Source: CAD feature listing. Evaluate the final solid. Frame: model axes, mm. A direction names the side the tool comes from. Round coordinates to 2 decimals unless told otherwise and drop trailing zeros. Loops run counter-clockwise (first coordinate to the right, second up) from the corner with the lowest first, then second, coordinate; pieces in that order, holes last. Notation, with made-up numbers: M 56,-19 L 101,-19 A12 ccw 101,2 Z; hole C 85.25,58 d6. An arc over 180 degrees is marked long. Answer as a JSON object with one key per item and string values.
Autodesk Inventor part; units mm, degrees
ref_plane "YZ Plane" through (0, 0, 0) normal (1, 0, 0) x (0, 1, 0)
ref_plane "XZ Plane" through (0, 0, 0) normal (0, 1, 0) x (-1, 0, 0)
ref_plane "XY Plane" through (0, 0, 0) normal (0, 0, 1) x (1, 0, 0)
sketch "Эскиз1" plane through (0, 0, 0) normal (0, 1, 0) x (-1, 0, 0)
  line L0 (-3.5, 0) -> (-3.5, -76)
  line L1 (0, 0) -> (0, -2)
  line L2 (0, -2) -> (0, -1)
  line L3 (0, -72) -> (0, -73)
  line L4 (0, 0) -> (0, -12)
  line L5 (0, -12) -> (8, -12)
  line L6 (8, -12) -> (56, -12)
  line L7 (56, -12) -> (62, -12)
  line L8 (62, -12) -> (62, -1)
  line L9 (62, -1) -> (0, -1)
  line L10 (0, -73) -> (62, -73)
  line L11 (62, -73) -> (62, -12)
  line L12 (0, -72) -> (62, -72)
  line L13 (0, -2) -> (62, -2)
  line L14 (3.5, -76) -> (3.5, 0)
  line L15 (0, 0) -> (3, 0)
  line L16 (3, 0) -> (3, 0.6)
  line L17 (56, -12) -> (68, -12)
  line L18 (68, -12) -> (73, -12)
  line L19 (8, -12) -> (10, -12)
  circle A0 centre (10, -12) radius 1.1
  circle A1 centre (68, -12) radius 1.1
  circle A2 centre (3, 0.6) radius 1.1
  circle A3 centre (3, 0.6) radius 3
  circle A4 centre (4, -76) radius 1.1
  circle A5 centre (4, -76) radius 3.5
  line L20 (7.5, -76) -> (7.5, -73)
  line L21 (0.5, -76) -> (0.5, -73)
  line L22 (0, -73) -> (-3.5, -73)
  line L23 (6, 0.6) -> (6, -1)
  line L24 (0, -1) -> (-3.5, -1)
  line L25 (62, -73) -> (73, -73)
  line L26 (73, -73) -> (73, -1)
  line L27 (73, -1) -> (62, -1)
  line L28 (62, -1) -> (62, -73)
  line L29 (0, 0.6) -> (0, 0)
  point P0 (3.5, -73)
  point P1 (0.0606, 0)
  dimension "d6" = 2
  dimension "d7" = 1
  dimension "d8" = 1
  dimension "d9" = 12
  dimension "d10" = 8
  dimension "d11" = 48
  dimension "d12" = 6
  dimension "d39" = 3
  dimension "d40" = 0.6
  dimension "d41" = 12
  dimension "d42" = 5
  dimension "d43" = 2
  dimension "d44" = 2.2
  dimension "d45" = 2.2
  dimension "d46" = 2.2
  dimension "d47" = 6
  dimension "d48" = 2.2
  dimension "d49" = 7
extrude "Выдавливание1" add sketch "Эскиз1" along normal blind 2 contours L24 L1 L4 L5 L14 L12 L3 L22 L0 | L9 A3 L13 L1 | L1 L15 A3 L9 | L3 L12 L14 A5 L10 | L29 A3 L15 | L13 A3 L14 L5 L4 | A3 L15 A2 L14 L9 | L9 L14 L13 A3 | L10 A5 L21 | A3 L9 L14 A2 L15 | L13 L14 A3 | L9 A3 L13 L14 | L14 L5 L6 A0 L7 L11 L12 | L12 L11 L10 A5 L14 | A5 L14 L10 | L10 A5 | L23 L9 A3 | L14 A3 L13 L8 L7 L6 A0 L5 | L13 A3 L14 | L9 L8 L13 A3 | L11 L17 A1 L18 L26 L25 | A5 L10 L14 | A5 L10 L20 | L8 L27 L26 L18 A1 L17
sketch "Эскиз2" plane through (0, 2, 0) normal (0, 1, 0) x (1, 0, 0)
  line L0 (-73, 1) -> (-6, 1)
  line L1 (3.5, 1) -> (3.5, 73)
  line L2 (-73, 1) -> (3.5, 1)
  line L3 (3.5, 1) -> (3.5, 2)
  line L4 (3.5, 2) -> (-73, 2)
  line L5 (-73, 2) -> (-73, 1)
  line L6 (-7.5, 73) -> (-73, 73)
  line L7 (-73, 73) -> (3.5, 73)
  line L8 (3.5, 73) -> (3.5, 72)
  line L9 (3.5, 72) -> (-73, 72)
  line L10 (-73, 72) -> (-73, 73)
  line L11 (0, 1) -> (3.5, 1)
  line L12 (3.5, 73) -> (1.5, 73)
  line L13 (1.5, 73) -> (1.5, 1)
  line L14 (1.5, 1) -> (3.5, 1)
  line L15 (3.5, 1) -> (3.5, 73)
  point P0 (-62, 73)
  point P1 (1.5, 72)
  point P2 (1.5, 2)
  dimension "d50" = 1
  dimension "d51" = 1
  dimension "d52" = 2
extrude "Выдавливание2" add sketch "Эскиз2" along normal blind 6
sketch "Эскиз3" plane through (-62, 0, -1) normal (0, 0, 1) x (1, 0, 0)
  line L0 (65.5, 8) -> (-11, 8)
  line L1 (65.5, 8) -> (43.5, 8)
  line L2 (63.5, 8) -> (54.5, 8)
  line L3 (54.5, 8) -> (54.5, 5)
  circle A0 centre (54.5, 5) radius 1.5
  line L4 (-11, 2) -> (63.5, 2)
  line L5 (43.5, 8) -> (-11, 2)
  line L6 (-11, 2) -> (-11, 8)
  line L7 (43.5, 8) -> (-11, 8)
  point P0 (65.5, 2)
  dimension "d53" = 22
  dimension "d54" = 9
  dimension "d55" = 3
  dimension "d56" = 3
extrude "Выдавливание3" cut sketch "Эскиз3" against normal blind 76
sketch "Эскиз4" plane through (0, 8, 0) normal (0, 1, 0) x (1, 0, 0)
  circle A0 centre (-3, -0.6) radius 1.1
  circle A1 centre (-3, -0.6) radius 2.1
  dimension "d57" = 4.2
extrude "Выдавливание4" cut sketch "Эскиз4" against normal blind 6 contours A0 | A1
chamfer "Фаска1" distance 1 angle 45 2 edges at (-8.9, 2, -12) (-66.9, 2, -12)
chamfer "Фаска2" distance 0.5 angle 45 2 edges at (-9, 5, -1) (-9, 5, -73)
sketch "Эскиз5" plane through (0, 0, 0) normal (0, -1, 0) x (1, 0, 0)
  line L0 (31.0823, 41.3034) -> (-105.9038, 41.3034)
  line L1 (-105.9038, 41.3034) -> (-105.9038, -112.9994)
  line L2 (-105.9038, -112.9994) -> (31.0823, -112.9994)
  line L3 (31.0823, -112.9994) -> (31.0823, 41.3034)
  point P0 (0, 0)
extrude "Выдавливание5" cut sketch "Эскиз5" against normal blind 0.5
properties part number "HDD"
Item 1: Line query: probe 1 along X at (y, z) = (0.95, -12); probe 2 along Y at (x, z) = (-7.5, -1.7); probe 3 along Z at (x, y) = (-20, 4.5). Output: solid intervals per line, ascending. Write a range as from..to.
Answer sheet:
{"probe 1": "x = -73..-69.1, -66.9..-11.1, -8.9..3.5", "probe 2": "y = 0.5..3.5, 6.5..8", "probe 3": "z = -73..-72, -2..-1"}
Item 2: Contact query for flat-ended pins moving along their axis: pin 1 Ø4 at (y, z) = (7, -31) entering from -X; pin 2 Ø5 at (x, z) = (-4.5, -77.5) entering from +Y; pin 3 Ø1.5 at (x, y) = (1.5, 4) entering from +Z. Output: stop coordinate, or through.
Answer sheet:
{"pin 1": "stops at x = 1.5", "pin 2": "stops at y = 2", "pin 3": "stops at z = -1"}
Item 3: Section B-B on z = -31.5. Return the cut outline in (x, y).
Answer sheet:
{"outline": "M -73,0.5 L 3.5,0.5 L 3.5,8 L 1.5,8 L 1.5,2 L -73,2 Z"}
Item 4: Pull-direction query (Z, two-part tool) for faces 1 (the cylindrical face through (-4.1, 1.2, -79.5)), 2 (the flat face through (-45.37, 5.04, -72.49)), 3 (the cylindrical face through (-4.016, 1.24, 1.021)), 4 (the flat face through (-35, 2, -37)); classes: pulls with the +Z half, pulls with the -Z half, needs draft (parallel to the pull), parting line crosses it, or undercut.
Answer sheet:
{"face 1": "pulls with the -Z half", "face 2": "needs draft", "face 3": "undercut", "face 4": "undercut"}
Item 5: Access query for faces 5 (the flat face through (-27, 4, -2)), 6 (the cylindrical face through (-3, 5, -1.5)), 7 (the flat face through (-5, 2, -77)). Directions: +Z, -Z, +X, -X, +Y, -Y. A direction counts if a zero-diameter tool reaches every point of the face in a straight line with its end or side. Return the directions, or none.
Answer sheet:
{"face 5": "-X, +Y", "face 6": "+Z, +Y", "face 7": "-Z, +X, -X, +Y"}
Item 6: Section A-A on x = -68. Return the cut outline in (y, z), then the cut area to 3 significant figures.
Answer sheet:
{"outline": "M 0.5,-73 L 2.55,-73 L 2.55,-72 L 2,-72 L 2,-14.1 L 1,-13.1 L 0.5,-13.1 Z; M 0.5,-10.9 L 1,-10.9 L 2,-9.9 L 2,-2 L 2.55,-2 L 2.55,-1 L 0.5,-1 Z", "area": "105 mm²"}
